The listing builds one solid part. Answer for the finished solid, in the listing's coordinates (mm). A direction names the side the tool comes from. Round coordinates to 2 decimals unless told otherwise and drop trailing zeros. Write each loop counter-clockwise with the first axis right and the second up, starting at its lowest first coordinate (ties: lowest second). Pieces come first, ordered by that corner, then holes.
from build123d import *

# Parameters (mm, degrees)
SCHIZZO1_W                        = 23
SCHIZZO1_H                        = 23
ESTRUSIONE_ESTRUSIONE1_DEPTH      = 55
TAGLIO_ESTRUSIONE12_REACH         = 60.671
SCHIZZO18_R                       = 7.1
SMUSSO4_SIZE                      = 1
SMUSSO4_SIZE2                     = 3
SCHIZZO19_R                       = 1.75
TAGLIO_ESTRUSIONE13_DEPTH         = 62.486055435
ESTRUSIONE_ESTRUSIONE2_REACH      = 63.486
ESTRUSIONE_ESTRUSIONE2_END_RADIUS = 7.1
SCHIZZO20_W                       = 2
SCHIZZO20_H                       = 3.5
ESTRUSIONE_ESTRUSIONE3_REACH      = 63.486
ESTRUSIONE_ESTRUSIONE3_END_RADIUS = 7.1
SCHIZZO21_W                       = 2
SCHIZZO21_H                       = 3.5
RACCORDO1_R                       = 3


with BuildPart() as part:
    # Schizzo1 → Estrusione-Estrusione1 (new body)
    with BuildSketch(Plane.XY):
        with Locations((-3.551080126, 2.313028552)):
            Rectangle(SCHIZZO1_W, SCHIZZO1_H)
    extrude(amount=ESTRUSIONE_ESTRUSIONE1_DEPTH)

    # Schizzo18 → Taglio-Estrusione12 (cut, up to next)
    with BuildSketch(Plane(origin=(0, 0, 0), x_dir=(-1, 0, 0), z_dir=(0, 0, -1)), mode=Mode.PRIVATE) as taglio_estrusione12_sk1:
        with Locations((3.551080126, 2.313028552)):
            Circle(SCHIZZO18_R)
    taglio_estrusione12_tool1 = extrude(taglio_estrusione12_sk1.sketch, amount=-TAGLIO_ESTRUSIONE12_REACH, mode=Mode.PRIVATE) & part.part
    add(taglio_estrusione12_tool1.solids().sort_by_distance((-3.55108, 2.313029, 0))[0], mode=Mode.SUBTRACT)

    # Smusso4
    smusso4_edges = [part.edges().sort_by_distance(p)[0] for p in [
        (3.548919874, 2.313028552, 0),
    ]]
    smusso4_side = [part.faces().sort_by_distance(p)[0] for p in [
        (-3.551080126, 13.487759433, 0),
    ]]
    chamfer(smusso4_edges, length=SMUSSO4_SIZE, length2=SMUSSO4_SIZE2, reference=smusso4_side[0])

    # Schizzo19 → Taglio-Estrusione13 (cut, through all)
    with BuildSketch(Plane(origin=(0, 13.813028552, 0), x_dir=(1, 0, 0), z_dir=(0, 1, 0))):
        with Locations(Location((-3.551080126, -50.55, 0), (0, 0, 180))):
            Circle(SCHIZZO19_R)
        with Locations(Location((-3.551080126, -9.45, 0), (0, 0, 180))):
            Circle(SCHIZZO19_R)
    extrude(amount=-TAGLIO_ESTRUSIONE13_DEPTH, mode=Mode.SUBTRACT)

    # Estrusione-Estrusione2: up to this cylinder (the profile starts outside it)
    estrusione_estrusione2_end = Plane(origin=(-3.551080126, 2.313028552, 30), z_dir=(0, 0, -1)) * Cylinder(ESTRUSIONE_ESTRUSIONE2_END_RADIUS, 183.272, mode=Mode.PRIVATE)
    # Schizzo20 → Estrusione-Estrusione2 (add, up to the surface)
    with BuildSketch(Plane(origin=(0, 13.813028552, 0), x_dir=(1, 0, 0), z_dir=(0, 1, 0)), mode=Mode.PRIVATE) as estrusione_estrusione2_sk1:
        with Locations((-3.551080126, -50.55)):
            Rectangle(SCHIZZO20_W, SCHIZZO20_H)
    estrusione_estrusione2_tool1 = extrude(estrusione_estrusione2_sk1.sketch, amount=-ESTRUSIONE_ESTRUSIONE2_REACH, mode=Mode.PRIVATE) - estrusione_estrusione2_end
    add(estrusione_estrusione2_tool1.solids().sort_by_distance((-3.55108, 13.813029, 50.55))[0])
    # Schizzo20 → Estrusione-Estrusione2 (add, up to the surface)
    with BuildSketch(Plane(origin=(0, 13.813028552, 0), x_dir=(1, 0, 0), z_dir=(0, 1, 0)), mode=Mode.PRIVATE) as estrusione_estrusione2_sk2:
        with Locations((-3.551080126, -9.45)):
            Rectangle(SCHIZZO20_W, SCHIZZO20_H)
    estrusione_estrusione2_tool2 = extrude(estrusione_estrusione2_sk2.sketch, amount=-ESTRUSIONE_ESTRUSIONE2_REACH, mode=Mode.PRIVATE) - estrusione_estrusione2_end
    add(estrusione_estrusione2_tool2.solids().sort_by_distance((-3.55108, 13.813029, 9.45))[0])

    # Estrusione-Estrusione3: up to this cylinder (the profile starts outside it)
    estrusione_estrusione3_end = Plane(origin=(-3.551080126, 2.313028552, 30), z_dir=(0, 0, -1)) * Cylinder(ESTRUSIONE_ESTRUSIONE3_END_RADIUS, 183.272, mode=Mode.PRIVATE)
    # Schizzo21 → Estrusione-Estrusione3 (add, up to the surface)
    with BuildSketch(Plane.XZ.offset(9.186971448), mode=Mode.PRIVATE) as estrusione_estrusione3_sk1:
        with Locations((-3.551080126, 9.45)):
            Rectangle(SCHIZZO21_W, SCHIZZO21_H)
    estrusione_estrusione3_tool1 = extrude(estrusione_estrusione3_sk1.sketch, amount=-ESTRUSIONE_ESTRUSIONE3_REACH, mode=Mode.PRIVATE) - estrusione_estrusione3_end
    add(estrusione_estrusione3_tool1.solids().sort_by_distance((-3.55108, -9.186971, 9.45))[0])
    # Schizzo21 → Estrusione-Estrusione3 (add, up to the surface)
    with BuildSketch(Plane.XZ.offset(9.186971448), mode=Mode.PRIVATE) as estrusione_estrusione3_sk2:
        with Locations((-3.551080126, 50.55)):
            Rectangle(SCHIZZO21_W, SCHIZZO21_H)
    estrusione_estrusione3_tool2 = extrude(estrusione_estrusione3_sk2.sketch, amount=-ESTRUSIONE_ESTRUSIONE3_REACH, mode=Mode.PRIVATE) - estrusione_estrusione3_end
    add(estrusione_estrusione3_tool2.solids().sort_by_distance((-3.55108, -9.186971, 50.55))[0])

    # Raccordo1
    raccordo1_edges = [part.edges().sort_by_distance(p)[0] for p in [
        (7.948919874, 13.813028552, 27.5),
        (7.948919874, -9.186971448, 27.5),
        (-15.051080126, -9.186971448, 27.5),
        (-15.051080126, 13.813028552, 27.5),
    ]]
    fillet(raccordo1_edges, radius=RACCORDO1_R)


solid = part.part
1. Section A-A on z = 9 is taken. Determine the outline of the cut face in (x, y), plus the area to 3 significant figures.
Geometry says:
outline: (-15.05, -6.19) arc R3 ccw to (-12.05, -9.19) - (-5.24, -9.19) - (-5.24, -4.58) arc R7.1 cw to (-5.24, 9.21) - (-5.24, 13.81) - (-12.05, 13.81) arc R3 ccw to (-15.05, 10.81) - close; (-4.55, -9.19) - (-2.55, -9.19) - (-2.55, -4.72) arc R7.1 cw to (-4.55, -4.72) - close; (-4.55, 9.34) arc R7.1 cw to (-2.55, 9.34) - (-2.55, 13.81) - (-4.55, 13.81) - close; (-1.86, -9.19) - (4.95, -9.19) arc R3 ccw to (7.95, -6.19) - (7.95, 10.81) arc R3 ccw to (4.95, 13.81) - (-1.86, 13.81) - (-1.86, 9.21) arc R7.1 cw to (-1.86, -4.58) - close
area: 350 mm2
2. Section C-C on x = 6 is taken. Determine the outline of the cut face in (y, z).
Geometry says:
outline: (-9, 0) - (13.62, 0) - (13.62, 55) - (-9, 55) - close
3. For a pull along X with two mould halves and no side action, classify faces 3 (the face through (-9, 8, 55)), 4 (the face through (-15.051, 2, 27)), 5 (the face through (-4.551, 12, 9)) as released by +X, released by -X, zero draft, split by the parting line, or undercut.
Geometry says:
face 3: zero draft
face 4: released by -X
face 5: undercut
4. Section B-B on z = 20.5 is taken. Determine the outline of the cut face in (x, y), plus the area to 3 significant figures.
Geometry says:
outline: (-15.05, -6.19) arc R3 ccw to (-12.05, -9.19) - (4.95, -9.19) arc R3 ccw to (7.95, -6.19) - (7.95, 10.81) arc R3 ccw to (4.95, 13.81) - (-12.05, 13.81) arc R3 ccw to (-15.05, 10.81) - close; hole circle Ø14.2 at (-3.55, 2.31)
area: 363 mm2
5. A tool of negligible diameter and unlimited length cuts with its end or side. For faces 1 (the face through (-4, 13.813, 27)), 2 (the face through (-4.551, -7, 9)), from which of +Z, -Z, +X, -X, +Y, -Y can it reach the whole face along a straight path? Write none if from no direction.
Geometry says:
face 1: +Z, -Z, +X, -X, +Y
face 2: +Y, -Y
6. Given pin 1 (0.9 mm diameter, centred on y = 11.5, z = 10, fed in from -X); pin 2 (1.4 mm diameter, centred on y = -8, z = 9.5, fed in from -X), each flat-ended and moving along its own axis, determine where each tip first touches the part or whether it passes through.
Geometry says:
pin 1: stops at x = -15.04
pin 2: stops at x = -14.84
7. Straight lines are drawn through the part: line 1 along X through (y, z) = (8.5, 5.5); line 2 along Y through (x, z) = (-4.75, 35.5); line 3 along Y through (x, z) = (-6.5, 23). For each, find the intervals that lie inside material, in ascending order.
Geometry says:
line 1: x = -15.05 to -7.03, -0.07 to 7.95
line 2: y = -9.19 to -4.69, 9.31 to 13.81
line 3: y = -9.19 to -4.15, 8.77 to 13.81
